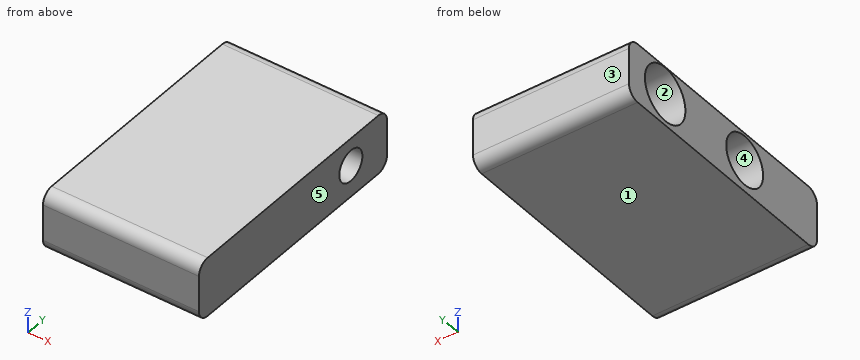
from build123d import *

# Parameters (mm, degrees)
SKETCH1_W           = 6.5
SKETCH1_H           = 26
SKETCH1_R           = 2.8
BOSS_EXTRUDE1_DEPTH = 16
SKETCH1_3_R         = 2.8
SKETCH1_3_R_2       = 1.6
BOSS_EXTRUDE3_DEPTH = 5
CUT_EXTRUDE2_START  = -16
SKETCH1_4_R         = 2.55
CUT_EXTRUDE2_DEPTH  = 8.4
CUT_EXTRUDE1_START  = 3.25
SKETCH2_R           = 50
CUT_EXTRUDE1_DEPTH  = 0.4
FILLET1_R           = 1.2


with BuildPart() as part:
    # Sketch1 → Boss-Extrude1 (new body)
    with BuildSketch(Plane(origin=(0, 0, 0), x_dir=(0, 0, -1), z_dir=(1, 0, 0))):
        with Locations((0, 8)):
            Rectangle(SKETCH1_W, SKETCH1_H)
        with Locations((0, 16)):
            Circle(SKETCH1_R, mode=Mode.SUBTRACT)
    extrude(amount=-BOSS_EXTRUDE1_DEPTH)

    # Sketch1<3> → Boss-Extrude3 (add)
    with BuildSketch(Plane(origin=(0, 0, 0), x_dir=(0, 0, -1), z_dir=(1, 0, 0))):
        with Locations((0, 16)):
            Circle(SKETCH1_3_R)
        with Locations((0, 16)):
            Circle(SKETCH1_3_R_2, mode=Mode.SUBTRACT)
    extrude(amount=-BOSS_EXTRUDE3_DEPTH)

    # Sketch1<4> → Cut-Extrude2 (cut)
    with BuildSketch(Plane(origin=(0, 0, 0), x_dir=(0, 0, -1), z_dir=(1, 0, 0)).offset(CUT_EXTRUDE2_START)):
        with Locations((0, 5)):
            Circle(SKETCH1_4_R)
    extrude(amount=CUT_EXTRUDE2_DEPTH, mode=Mode.SUBTRACT)

    # Sketch2 → Cut-Extrude1 (cut)
    with BuildSketch(Plane.XY.offset(CUT_EXTRUDE1_START)):
        Circle(SKETCH2_R)
    extrude(amount=-CUT_EXTRUDE1_DEPTH, mode=Mode.SUBTRACT)

    # Fillet1
    fillet1_edges = [part.edges().sort_by_distance(p)[0] for p in [
        (-8, 21, -3.25),
        (-8, -5, -3.25),
        (-8, 21, 2.85),
        (-8, -5, 2.85),
    ]]
    fillet(fillet1_edges, radius=FILLET1_R)


solid = part.part
Could you check a few things on this model? Use its own coordinates, in mm. Face numbers are marked on the shaded views. A direction names the side the tool comes from. Give positions to 0.01 mm unless a question says otherwise; leave off trailing zeros. Write each loop counter-clockwise with the first axis right and the second up, starting at its lowest first coordinate (ties: lowest second). Pieces come first, ordered by that corner, then holes. Notation, with made-up numbers: (-10.75, 17.5) -> (31.25, 17.5) arc R11 ccw to (31.25, 24.5) -> close; hole circle Ø1 at (45, 39.5). An arc over 180 degrees is marked (long way). Answer as CSV lines item,"result". Start each with the question number.
(1) Please list where these lines run through material, in increasing order: line 1 (Y direction, x = -10.5, z = 0); line 2 (Y direction, x = -12.75, z = 2); line 3 (Y direction, x = -2.55, z = 0).
(2) If we section it at D-D, the plane y = 5: Write out the boundary of the cut face in (x, z), and give its area (3 significant figures).
(3) If we section it at A-A, the plane y = 16: Write out the boundary of the cut face in (x, z), and give its area (3 significant figures).
(4) Which directions (+Z, -Z, +X, -X, +Y, -Y) give clear straight access to the entire face, cutting with the end or side of a thin tool? Please do the marked faces 4 and 5.
(5) If we section it at B-B, the plane z = 0: Write out the boundary of the cut face in (x, y).
(6) If we mould it in two halves opening along Z, with no side actions, what happens to the marked faces 1, 2 and 3? For each: +Z half, -Z half, draft (parallel to the pull), parting line (faces both ways), or undercut.
(7) I'm going to push a flat-ended pin straight in: pin 1 Ø3 at (y, z) = (5, 0) entering from +X. Where does the tip first touch, or does it pass through?
(8) If we section it at C-C, the plane x = -3.25: Write out the boundary of the cut face in (y, z).
Answer list:
1,line 1,"-5 to 2.45, 7.55 to 13.2, 18.8 to 21"
1,line 2,"-4.95 to 3.42, 6.58 to 14.04, 17.96 to 20.95"
1,line 3,"-5 to 14.4, 17.6 to 21"
2,outline,"(-16, -3.25) -> (0, -3.25) -> (0, 2.85) -> (-16, 2.85) -> (-16, 2.55) -> (-7.6, 2.55) -> (-7.6, -2.55) -> (-16, -2.55) -> close"
2,area,"54.8 mm^2"
3,outline,"(-16, -3.25) -> (0, -3.25) -> (0, -1.6) -> (-5, -1.6) -> (-5, -2.8) -> (-16, -2.8) -> close; (-16, 2.8) -> (-5, 2.8) -> (-5, 1.6) -> (0, 1.6) -> (0, 2.85) -> (-16, 2.85) -> close"
3,area,"20.0 mm^2"
4,face 4,"-X"
4,face 5,"+Z, -Z, +X, +Y, -Y"
5,outline,"(-16, -5) -> (0, -5) -> (0, 14.4) -> (-5, 14.4) -> (-5, 13.2) -> (-16, 13.2) -> (-16, 7.55) -> (-7.6, 7.55) -> (-7.6, 2.45) -> (-16, 2.45) -> close; (-16, 18.8) -> (-5, 18.8) -> (-5, 17.6) -> (0, 17.6) -> (0, 21) -> (-16, 21) -> close"
6,face 1,"-Z half"
6,face 2,"undercut"
6,face 3,"draft"
7,pin 1,"x = 0"
8,outline,"(-5, -2.05) arc R1.2 ccw to (-3.8, -3.25) -> (19.8, -3.25) arc R1.2 ccw to (21, -2.05) -> (21, 1.65) arc R1.2 ccw to (19.8, 2.85) -> (-3.8, 2.85) arc R1.2 ccw to (-5, 1.65) -> close; hole circle Ø3.2 at (16, 0)"
